```python
from build123d import *

# Parameters (mm, degrees)
SKETCH1_R                = 2.1717
BOSS_EXTRUDE1_DEPTH      = 2.54
BOSS_EXTRUDE2_DEPTH      = 25.4
BOSS_EXTRUDE2_DEPTH_BACK = 2.54
SKETCH2_W                = 10.16
SKETCH2_H                = 7.62
SKETCH3_W                = 5.08
SKETCH3_H                = 4.597654895
BOSS_EXTRUDE3_DEPTH      = 12.7
BOSS_EXTRUDE4_DEPTH      = 5.08


with BuildPart() as part:
    # Sketch1 → Boss-Extrude1 (new body)
    with BuildSketch(Plane(origin=(0, 0, 0), x_dir=(1, 0, 0), z_dir=(0, 1, 0))):
        Polygon((0, -5.08), (-5.08, -5.08), (-5.08, 4.572), (5.08, 4.572), (13.309339364, -5.08), (48.607458274, -5.08), (55.88, 4.572), (66.04, 4.572), (66.04, -5.08), (60.96, -5.08), (55.88, -5.08), (51.60608488, -9.677654895), (10.567737895, -9.677654895), (5.08, -5.08), align=None)
        with Locations(Location((0, 0, 0), (0, 0, 270))):
            Circle(SKETCH1_R, mode=Mode.SUBTRACT)
        with Locations(Location((60.96, 0, 0), (0, 0, 270))):
            Circle(SKETCH1_R, mode=Mode.SUBTRACT)
    extrude(amount=BOSS_EXTRUDE1_DEPTH)

    # Sketch2 → Boss-Extrude2 (add, two sides: drawn at the far end of the back side and taken through both)
    with BuildSketch(Plane(origin=(0, 2.54, 0), x_dir=(1, 0, 0), z_dir=(0, 1, 0)).offset(-BOSS_EXTRUDE2_DEPTH_BACK)):
        with Locations((0, -8.89)):
            Rectangle(SKETCH2_W, SKETCH2_H)
    extrude(amount=BOSS_EXTRUDE2_DEPTH + BOSS_EXTRUDE2_DEPTH_BACK)

    # Sketch3 → Boss-Extrude3 (add)
    with BuildSketch(Plane(origin=(0, 2.54, 0), x_dir=(1, 0, 0), z_dir=(0, 1, 0))):
        with Locations((34.036, -7.378827447)):
            Rectangle(SKETCH3_W, SKETCH3_H)
    extrude(amount=BOSS_EXTRUDE3_DEPTH)

    # Sketch4 → Boss-Extrude4 (add)
    with BuildSketch(Plane(origin=(36.576, 0, 0), x_dir=(0, 0, -1), z_dir=(1, 0, 0))):
        Polygon((-5.08, 15.24), (2.54, 15.24), (2.54, 10.026233787), (0, 10.026233787), (0, 12.566233787), (-5.08, 12.566233787), align=None)
    extrude(amount=-BOSS_EXTRUDE4_DEPTH)


solid = part.part
```
CAD build for the part. Positions are in the model's coordinates, mm. A direction names the side the tool comes from. Round coordinates to 2 decimals unless told otherwise and drop trailing zeros. Order: outer loops, then holes, each group sorted by start corner. A loop starts at its lowest first (then second) coordinate and runs counter-clockwise, first axis right, second up.
Q1. Two-plate mould, pull along Z, no slides. Class faces 1 (the flat face through (-5.08, 14, 8)), 2 (the flat face through (34, 12.566, 3)), 3 (the flat face through (0, 14, 12.7)), 4 (the cylindrical face through (0.652, 1.252, 2.071)): pulls with the +Z half, pulls with the -Z half, needs draft (parallel to the pull), parting line crosses it, or undercut.
Q2. Slice it at D-D (x = 33.5). Write the cut outline in (y, z), and give its area (3 significant figures).
Q3. Slice it at C-C (z = -0.75). Write the cut outline in (x, y), and give its area (3 significant figures).
Q4. Slice it at B-B (y = 14). Write the cut outline in (x, z).
Q5. Wall check: L1, parallel to X at y = 1.95, z = 0; L2, parallel to Z at x = 1, y = 7.75; L3, parallel to X at y = 12.25, z = 10.5. Give the ranges that are in metal, low to high.
Q6. Which spindle directions (+Z, -Z, +X, -X, +Y, -Y) get a long thin tool onto all of the face, cutting with end or side? Do faces 5 (the flat face through (34, 15.24, 4)), 6 (the flat face through (31.496, 10, 6)), 7 (the flat face through (9, 2.54, 4)). Say none if no direction does.
Q7. Slice it at A-A (x = 60.96). Write the cut outline in (y, z), and give its area (3 significant figures).
Q8. Drop flat-ended pins along their axis: pin 1 (3 mm diameter, centred on x = 6, y = 20, fed in from -Z); pin 2 (5.5 mm diameter, centred on x = 33, z = 1, fed in from +Y); pin 3 (0.8 mm diameter, centred on x = 61, y = 1, fed in from +Z); pin 4 (5.5 mm diameter, centred on x = 33, z = 3.5, fed in from -Y). Give the stop position or say it passes through.
Results below:
1. face 1: needs draft
1. face 2: undercut
1. face 3: pulls with the +Z half
1. face 4: undercut
2. outline: (0, 5.08) - (12.57, 5.08) - (12.57, 0) - (10.03, 0) - (10.03, -2.54) - (15.24, -2.54) - (15.24, 9.68) - (0, 9.68) - close
2. area: 96.9 mm2
3. outline: (-5.08, 0) - (-2.04, 0) - (-2.04, 2.54) - (-5.08, 2.54) - close; (2.04, 0) - (8.34, 0) - (8.34, 2.54) - (2.04, 2.54) - close; (31.5, 10.03) - (36.58, 10.03) - (36.58, 15.24) - (31.5, 15.24) - close; (53, 0) - (58.92, 0) - (58.92, 2.54) - (53, 2.54) - close; (63, 0) - (66.04, 0) - (66.04, 2.54) - (63, 2.54) - close
3. area: 73.0 mm2
4. outline: (-5.08, 5.08) - (5.08, 5.08) - (5.08, 12.7) - (-5.08, 12.7) - close; (31.5, -2.54) - (36.58, -2.54) - (36.58, 9.68) - (31.5, 9.68) - close
5. L1: x = -5.08 to -2.17, 2.17 to 8.98, 52.44 to 58.79, 63.13 to 66.04
5. L2: z = 5.08 to 12.7
5. L3: x = -5.08 to 5.08
6. face 5: +Z, -Z, +X, +Y
6. face 6: +Z, -Z, +Y
6. face 7: -Z, +Y
7. outline: (0, -4.57) - (2.54, -4.57) - (2.54, -2.17) - (0, -2.17) - close; (0, 2.17) - (2.54, 2.17) - (2.54, 5.08) - (0, 5.08) - close
7. area: 13.5 mm2
8. pin 1: stops at z = 5.08
8. pin 2: stops at y = 15.24
8. pin 3: stops at z = 5.08
8. pin 4: stops at y = 0
